Could you check a few things on this drawing? It's one solid part, dimensions in mm from its lowest x, y, z. A direction names the side the tool comes from. Coordinates: 2 decimals unless noted, no trailing zeros. Loops run counter-clockwise (first coordinate to the right, second up) from the corner with the lowest first, then second, coordinate; pieces in that order, holes last. Notation, with made-up numbers: (-25, 53) -> (15, 53) arc R20 cw to (15, 74) -> close; hole circle Ø7 at (-21, 23.25). An arc over 180 degrees is marked (long way). One line per question, with ' | ' between items.
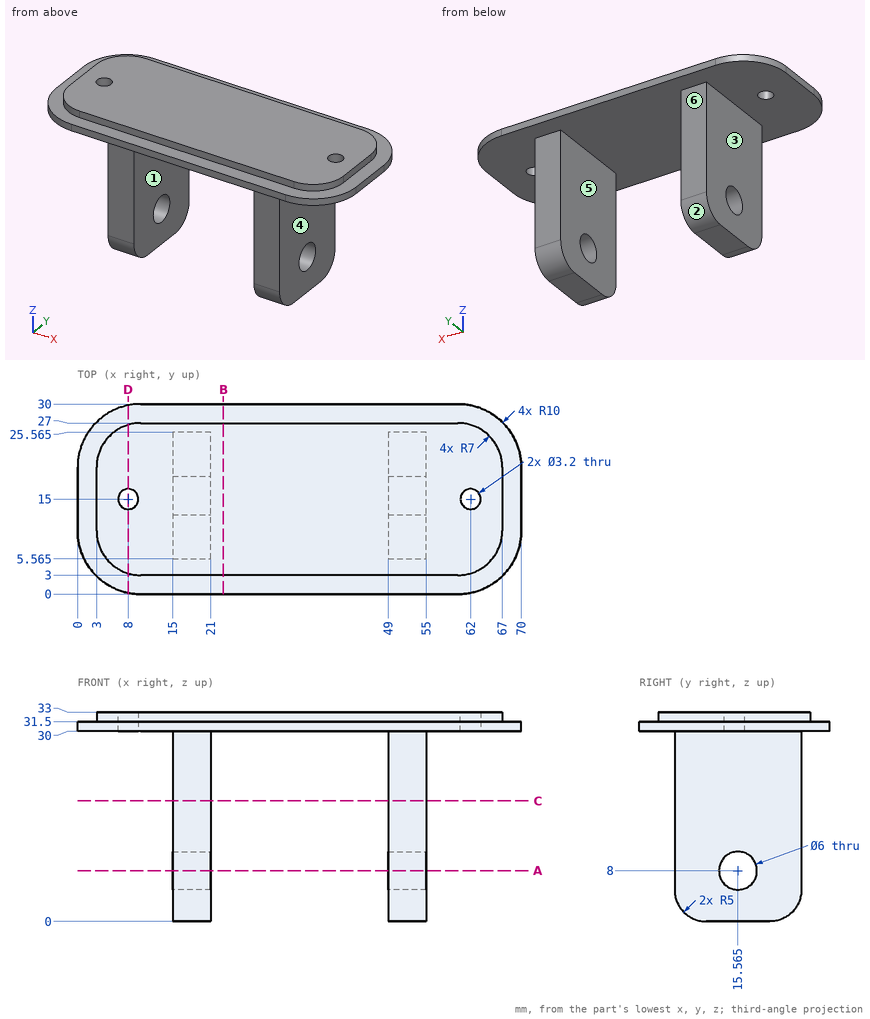
1) On a 3-axis mill with a long thin cutter (end or side, diameter ignored), from which of +Z, -Z, +X, -X, +Y, -Y can I reach the whole of each face in a straight line? I mean the marked faces 4, 5 and 6. Say none if no direction works.
Data:
face 4: -Z, +X, +Y, -Y | face 5: -Z, +Y, -Y | face 6: -Z, +X, -X, +Y
2) If we section it at A-A on z = 8: Please give me the cut outline in (x, y) (1 decimal).
Data:
outline: (15, 5.6) -> (21, 5.6) -> (21, 12.6) -> (15, 12.6) -> close; (15, 18.6) -> (21, 18.6) -> (21, 25.6) -> (15, 25.6) -> close; (49, 5.6) -> (55, 5.6) -> (55, 12.6) -> (49, 12.6) -> close; (49, 18.6) -> (55, 18.6) -> (55, 25.6) -> (49, 25.6) -> close
3) I'm going to push flat-ended pins straight in: pin 1 Ø1.8 at (x, z) = (52, 18.5) entering from -Y (1 decimal); pin 2 Ø5 at (x, z) = (26.5, 26) entering from +Y; pin 3 Ø5 at (y, z) = (26, 20.5) entering from -X; pin 4 Ø1.6 at (y, z) = (15.5, 32) entering from -X. Where does each tip first touch, or does it pass through?
Data:
pin 1: y = 5.6 | pin 2: through | pin 3: x = 15 | pin 4: x = 0
4) We'd pull the mould along X, two halves only. Please class the marked faces 1, 2 and 3: pulls with the +X half, pulls with the -X half, needs draft (parallel to the pull), parting line crosses it, or undercut.
Data:
face 1: undercut | face 2: needs draft | face 3: pulls with the -X half
5) I need wall thicknesses on line 1 along X through (y, z) = (17, 14); line 2 along Y through (x, z) = (50.45, 8) (1 decimal); line 3 along Z through (x, y) = (17.5, 15.75) (1 decimal). Which ranges of each line are inside material? Lowest first, please. Write a range as from..to.
Data:
line 1: 15..21, 49..55 | line 2: 5.6..12.6, 18.6..25.6 | line 3: 0..5, 11..33
6) If we section it at C-C on z = 19: Please give me the cut outline in (x, y) (1 decimal).
Data:
outline: (15, 5.6) -> (21, 5.6) -> (21, 25.6) -> (15, 25.6) -> close; (49, 5.6) -> (55, 5.6) -> (55, 25.6) -> (49, 25.6) -> close
7) If we section it at B-B on x = 23: Please give me the cut outline in (y, z).
Data:
outline: (0, 30) -> (30, 30) -> (30, 31.5) -> (27, 31.5) -> (27, 33) -> (3, 33) -> (3, 31.5) -> (0, 31.5) -> close
8) If we section it at D-D on x = 8: Please give me the cut outline in (y, z).
Data:
outline: (0.2, 30) -> (13.4, 30) -> (13.4, 33) -> (3.29, 33) -> (3.29, 31.5) -> (0.2, 31.5) -> close; (16.6, 30) -> (29.8, 30) -> (29.8, 31.5) -> (26.71, 31.5) -> (26.71, 33) -> (16.6, 33) -> close
